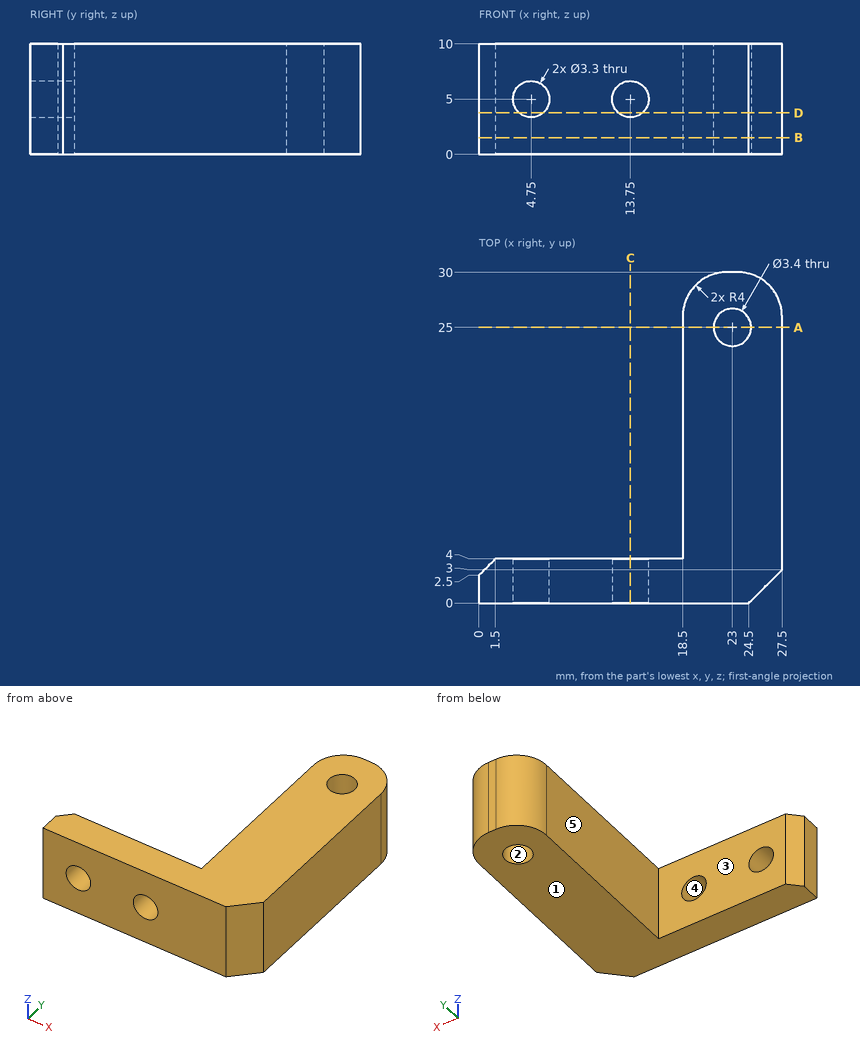
Print and shaded views of the part. All mm, measured from the part's lowest x, y and z. A direction names the side the tool comes from. Give positions to 0.01 mm unless a question says otherwise; leave off trailing zeros. Write each loop counter-clockwise with the first axis right and the second up, starting at its lowest first coordinate (ties: lowest second). Pieces come first, ordered by that corner, then holes. Notation, with made-up numbers: (82.25, -3.75) -> (101.25, -3.75) arc R9 ccw to (101.25, 5.25) -> close; hole circle Ø6 at (21, 10). An arc over 180 degrees is marked (long way). Use CSV: the item, a comma, the result in double quotes. Start each with the question number.
1) Cut at C-C on x = 13.75. List the corners of the cut face in (y, z).
2) Drill centre lines: L1, parallel to Z at x = 4.75, y = 2.95; L2, parallel to Y at x = 23, z = 3.25; L3, parallel to Y at x = 4, z = 9.75. Where is each one in solid material? Low to high.
3) Cut at D-D on z = 3.75. List the corners of the cut face in (x, y).
4) Tool access for the marked faces 4 and 5: list every direction of +Z, -Z, +X, -X, +Y, -Y with a clear straight run to the whole face (end or side of a thin tool).
5) Pin check, flat tips, straight feed: P1, Ø5.5, axis at x = 4.75, z = 5, coming from the +Y side; P2, Ø2, axis at y = 16, z = 2.5, coming from the -X side. Stop position of each tip, or through.
6) Two-plate mould, pull along Y, no slides. Class the marked faces 1, 2 and 3: released by +Y, released by -Y, zero draft, split by the parting line, or undercut.
7) Cut at A-A on y = 25. List the corners of the cut face in (x, z), plus the area to 3 significant figures.
8) Cut at B-B on z = 1.5. List the corners of the cut face in (x, y).
Final values:
1,outline,"(0, 0) -> (4, 0) -> (4, 3.35) -> (0, 3.35) -> close; (0, 6.65) -> (4, 6.65) -> (4, 10) -> (0, 10) -> close"
2,L1,"z = 0 to 3.35, 6.65 to 10"
2,L2,"y = 0 to 23.3, 26.7 to 30"
2,L3,"y = 0 to 4"
3,outline,"(0, 0) -> (3.67, 0) -> (3.67, 4) -> (1.5, 4) -> (0, 2.5) -> close; (5.83, 0) -> (12.67, 0) -> (12.67, 4) -> (5.83, 4) -> close; (14.83, 0) -> (24.5, 0) -> (27.5, 3) -> (27.5, 26) arc R4 ccw to (23.5, 30) -> (22.5, 30) arc R4 ccw to (18.5, 26) -> (18.5, 4) -> (14.83, 4) -> close; hole circle Ø3.4 at (23, 25)"
4,face 4,"+Y, -Y"
4,face 5,"+Z, -Z, -X, +Y"
5,P1,"stops at y = 4"
5,P2,"stops at x = 18.5"
6,face 1,"zero draft"
6,face 2,"undercut"
6,face 3,"released by +Y"
7,outline,"(18.5, 0) -> (21.3, 0) -> (21.3, 10) -> (18.5, 10) -> close; (24.7, 0) -> (27.5, 0) -> (27.5, 10) -> (24.7, 10) -> close"
7,area,"56.0 mm2"
8,outline,"(0, 0) -> (24.5, 0) -> (27.5, 3) -> (27.5, 26) arc R4 ccw to (23.5, 30) -> (22.5, 30) arc R4 ccw to (18.5, 26) -> (18.5, 4) -> (1.5, 4) -> (0, 2.5) -> close; hole circle Ø3.4 at (23, 25)"
